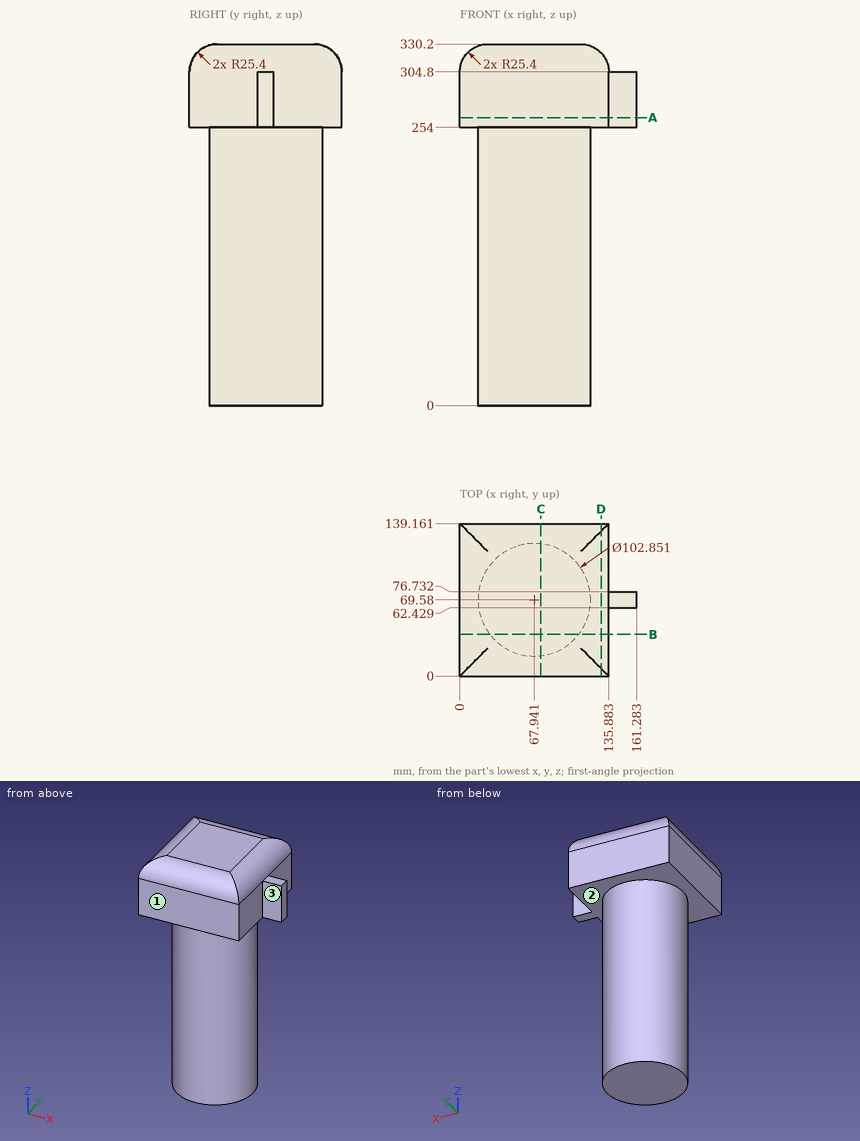
For this review, use the dimensioned drawing (mm, ordinates from the lowest corner) and the shaded views. A direction names the side the tool comes from. Give positions to 0.01 mm unless a question says otherwise; leave off trailing zeros. Order: outer loops, then holes, each group sorted by start corner. A loop starts at its lowest first (then second) coordinate and runs counter-clockwise, first axis right, second up. Notation, with made-up numbers: (-15.75, 89) -> (18.25, 89) arc R29 ccw to (18.25, 111) -> close; hole circle Ø9 at (-19, -30.75). An arc over 180 degrees is marked (long way). Write item = value, one per line. Start each with the question number.
(1) For pin 1 Ø20.5 at (x, z) = (148.5, 284) entering from +Y; pin 2 Ø10 at (x, z) = (106, 186.5) entering from +Y; pin 3 Ø1 at (x, z) = (88.5, 173.5) entering from -Y, all flat-tipped, find the tip position at first contact; note any pin that passes through.
(2) Take a section at D-D (x = 129). Write out the cut boundary in (y, z), plus the area to 3 significant figures.
(3) Tool access review of the marked faces 1, 2 and 3: name each direction out of +Z, -Z, +X, -X, +Y, -Y from which nothing blocks a thin tool from reaching the whole face with its end or side.
(4) Take a section at C-C (x = 74). Write out the cut boundary in (y, z).
(5) For L1, parallel to X at y = 72, z = 60.5; L2, parallel to Y at x = 70, z = 93.5 (1 decimal); L3, parallel to X at y = 23.5, z = 258.5, list the stretches that pass through material, from the lowest coordinate up. Write a range as from..to.
(6) Take a section at B-B (y = 38). Write out the cut boundary in (x, z) (1 decimal).
(7) Take a section at A-A (z = 263). Write out the cut boundary in (x, y), plus the area to 3 significant figures.
Returned:
q1.pin_1 = 76.73
q1.pin_2 = 108.97
q1.pin_3 = 22.23
q2.outline = (0, 254) -> (139.16, 254) -> (139.16, 304.8) arc R25.4 ccw to (132.28, 322.19) -> (6.88, 322.19) arc R25.4 ccw to (0, 304.8) -> close
q2.area = 9,410 mm²
q3.face_1 = +Z, -Z, +X, -X, -Y
q3.face_2 = -Z
q3.face_3 = +Z, -Z, +X, -Y
q4.outline = (0, 254) -> (18.51, 254) -> (18.51, 0) -> (120.65, 0) -> (120.65, 254) -> (139.16, 254) -> (139.16, 304.8) arc R25.4 ccw to (113.76, 330.2) -> (25.4, 330.2) arc R25.4 ccw to (0, 304.8) -> close
q5.L1 = 16.57..119.31
q5.L2 = 18.2..121
q5.L3 = 0..135.88
q6.outline = (0, 254) -> (27.4, 254) -> (27.4, 0) -> (108.5, 0) -> (108.5, 254) -> (135.9, 254) -> (135.9, 304.8) arc R25.4 ccw to (110.5, 330.2) -> (25.4, 330.2) arc R25.4 ccw to (0, 304.8) -> close
q7.outline = (0, 0) -> (135.88, 0) -> (135.88, 62.43) -> (161.28, 62.43) -> (161.28, 76.73) -> (135.88, 76.73) -> (135.88, 139.16) -> (0, 139.16) -> close
q7.area = 19,300 mm²
